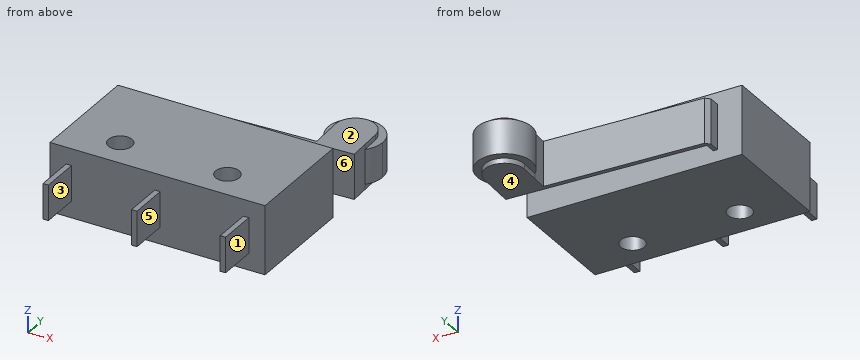
```python
from build123d import *

# Parameters (mm, degrees)
F0_R          = 1.1
F1_DEPTH      = 3.175
F1_DEPTH_BACK = 3.175
F2_DEPTH      = 2.075
F2_DEPTH_BACK = 2.075
F0_W          = 0.5
F0_H          = 3.63
F3_DEPTH      = 1.635
F3_DEPTH_BACK = 1.635
F4_DEPTH      = 1.6
F4_DEPTH_BACK = 1.6


with BuildPart() as f1:
    # F0 (on Top) → F1 (new body, two sides)
    with BuildSketch(Plane.XY) as f1_sk:
        Polygon((8.45, -5.32), (9.95, -5.32), (9.95, 5.32), (0, 5.32), (-7.28, 5.32), (-7.68, 5.32), (-9.95, 5.32), (-9.95, -5.32), (-8.45, -5.32), (-7.95, -5.32), (-0.25, -5.32), (0.25, -5.32), (7.95, -5.32), align=None)
        with Locations((-5.1, -2.52)):
            Circle(F0_R, mode=Mode.SUBTRACT)
        with Locations((4.82, -2.52)):
            Circle(F0_R, mode=Mode.SUBTRACT)
    extrude(amount=F1_DEPTH)
    extrude(f1_sk.sketch, amount=-F1_DEPTH_BACK)

    # F0 (on Top) → F2 (join, two sides)
    with BuildSketch(Plane.XY) as f2_sk:
        with BuildLine():
            Line((-7.68, 5.32), (-7.28, 5.32))
            Line((-7.28, 5.32), (-7.28, 6.32))
            Line((-7.28, 6.32), (10.906001, 7.033709))
            Line((10.906001, 7.033709), (10.835264, 8.836148))
            ThreePointArc((10.835264, 8.836148), (9.056806, 7.996935), (7.218048, 8.69419))
            Line((7.218048, 8.69419), (7.273099, 7.291444))
            Line((7.273099, 7.291444), (-7.295686, 6.719692))
            Line((-7.295686, 6.719692), (-7.68, 6.32))
            Line((-7.68, 6.32), (-7.68, 5.32))
        make_face()
        with BuildLine():
            ThreePointArc((7.218048, 8.69419), (9.056806, 7.996935), (10.835264, 8.836148))
            Line((10.835264, 8.836148), (10.766788, 10.580979))
            ThreePointArc((10.766788, 10.580979), (8.887202, 12.318608), (7.149573, 10.439021))
            Line((7.149573, 10.439021), (7.218048, 8.69419))
        make_face()
    extrude(amount=F2_DEPTH)
    extrude(f2_sk.sketch, amount=-F2_DEPTH_BACK)

    # F0 (on Top) → F3 (join, two sides)
    with BuildSketch(Plane.XY) as f3_sk:
        with Locations((-8.2, -7.135)):
            Rectangle(F0_W, F0_H)
        with Locations((8.2, -7.135)):
            Rectangle(F0_W, F0_H)
        with Locations((0, -7.135)):
            Rectangle(F0_W, F0_H)
    extrude(amount=F3_DEPTH)
    extrude(f3_sk.sketch, amount=-F3_DEPTH_BACK)

    # F0 (on Top) → F4 (join, two sides)
    with BuildSketch(Plane.XY) as f4_sk:
        with BuildLine():
            Line((10.766788, 10.580979), (10.835264, 8.836148))
            ThreePointArc((10.835264, 8.836148), (11.308296, 9.614355), (11.47318, 10.51))
            ThreePointArc((11.47318, 10.51), (7.971065, 12.823186), (7.218048, 8.69419))
            Line((7.218048, 8.69419), (7.149573, 10.439021))
            ThreePointArc((7.149573, 10.439021), (8.887202, 12.318608), (10.766788, 10.580979))
        make_face()
    extrude(amount=F4_DEPTH)
    extrude(f4_sk.sketch, amount=-F4_DEPTH_BACK)


solid = f1.part
```
Work out the finished part from the listing and answer in its coordinate system (mm). Face numbers are marked on the shaded views. A direction names the side the tool comes from. Coordinates: 2 decimals unless noted, no trailing zeros. Write each loop counter-clockwise with the first axis right and the second up, starting at its lowest first coordinate (ties: lowest second). Pieces come first, ordered by that corner, then holes. Notation, with made-up numbers: (-26, 7.25) - (2, 7.25) arc R8 ccw to (2, 22.25) - close; hole circle Ø9 at (51, 55.25). An arc over 180 degrees is marked (long way). Answer as a JSON object with one key per item and string values.
Q1. Given pin 1 Ø2 at (x, y) = (8.5, 11.5) entering from -Z (3 decimals); pin 2 Ø1.5 at (x, z) = (-7.5, -2.5) entering from +Y; pin 3 Ø0.6 at (x, y) = (8, -7) entering from +Z (3 decimals), each flat-ended and moving along its own axis, determine where each tip first touches the part or whether it passes through.
Results list:
{"pin 1": "stops at z = -2.075", "pin 2": "stops at y = 6.74", "pin 3": "stops at z = 1.635"}
Q2. For a pull along Y with two mould halves and no side action, classify the marked faces 5 and 6 as pulls with the +Y half, pulls with the -Y half, needs draft (parallel to the pull), parting line crosses it, or undercut.
Results list:
{"face 5": "needs draft", "face 6": "undercut"}
Q3. Find section A-A (y = -2.52). Write down the section's boundary in (x, z) (3 decimals), plus the area to 3 significant figures.
Results list:
{"outline": "(-9.95, -3.175) - (-6.2, -3.175) - (-6.2, 3.175) - (-9.95, 3.175) - close; (-4, -3.175) - (3.72, -3.175) - (3.72, 3.175) - (-4, 3.175) - close; (5.92, -3.175) - (9.95, -3.175) - (9.95, 3.175) - (5.92, 3.175) - close", "area": "98.4 mm^2"}
Q4. Find section D-D (x = -5.5). Write down the section's boundary in (y, z) (3 decimals), plus the area to 3 significant figures.
Results list:
{"outline": "(-5.32, -3.175) - (-3.545, -3.175) - (-3.545, 3.175) - (-5.32, 3.175) - close; (-1.495, -3.175) - (5.32, -3.175) - (5.32, 3.175) - (-1.495, 3.175) - close; (6.39, -2.075) - (6.79, -2.075) - (6.79, 2.075) - (6.39, 2.075) - close", "area": "56.2 mm^2"}
Q5. Find section B-B (x = -1.5). Write down the section's boundary in (y, z) (3 decimals), plus the area to 3 significant figures.
Results list:
{"outline": "(-5.32, -3.175) - (5.32, -3.175) - (5.32, 3.175) - (-5.32, 3.175) - close; (6.547, -2.075) - (6.947, -2.075) - (6.947, 2.075) - (6.547, 2.075) - close", "area": "69.2 mm^2"}
Q6. Find section C-C (z = 0.5). Write down the section's boundary in (x, y) (3 decimals).
Results list:
{"outline": "(-9.95, -5.32) - (-8.45, -5.32) - (-8.45, -8.95) - (-7.95, -8.95) - (-7.95, -5.32) - (-0.25, -5.32) - (-0.25, -8.95) - (0.25, -8.95) - (0.25, -5.32) - (7.95, -5.32) - (7.95, -8.95) - (8.45, -8.95) - (8.45, -5.32) - (9.95, -5.32) - (9.95, 5.32) - (-7.28, 5.32) - (-7.28, 6.32) - (10.906, 7.034) - (10.835, 8.836) arc R2.515 ccw (long way) to (7.218, 8.694) - (7.273, 7.291) - (-7.296, 6.72) - (-7.68, 6.32) - (-7.68, 5.32) - (-9.95, 5.32) - close; hole circle Ø2.2 at (-5.1, -2.52); hole circle Ø2.2 at (4.82, -2.52)"}
Q7. Consider L1, parallel to Y at x = -5.1, z = 2.25; L2, parallel to Y at x = -4.75, z = -0.25; L3, parallel to Y at x = -5.1, z = 1. Determine where each line is inside the solid, lowest interval first. Write a range as from..to.
Results list:
{"L1": "y = -5.32..-3.62, -1.42..5.32", "L2": "y = -5.32..-3.56, -1.48..5.32, 6.42..6.82", "L3": "y = -5.32..-3.62, -1.42..5.32, 6.41..6.81"}
Q8. Which of the six approach directions +Z, -Z, +X, -X, +Y, -Y give full straight-line access (tool end or side, diameter ignored) to the marked faces 1, 2, 3 and 4?
Results list:
{"face 1": "+Z, -Z, +X, -Y", "face 2": "+Z, +X, -X, +Y", "face 3": "+Z, -Z, -Y", "face 4": "-Z, +X, -X, +Y"}
